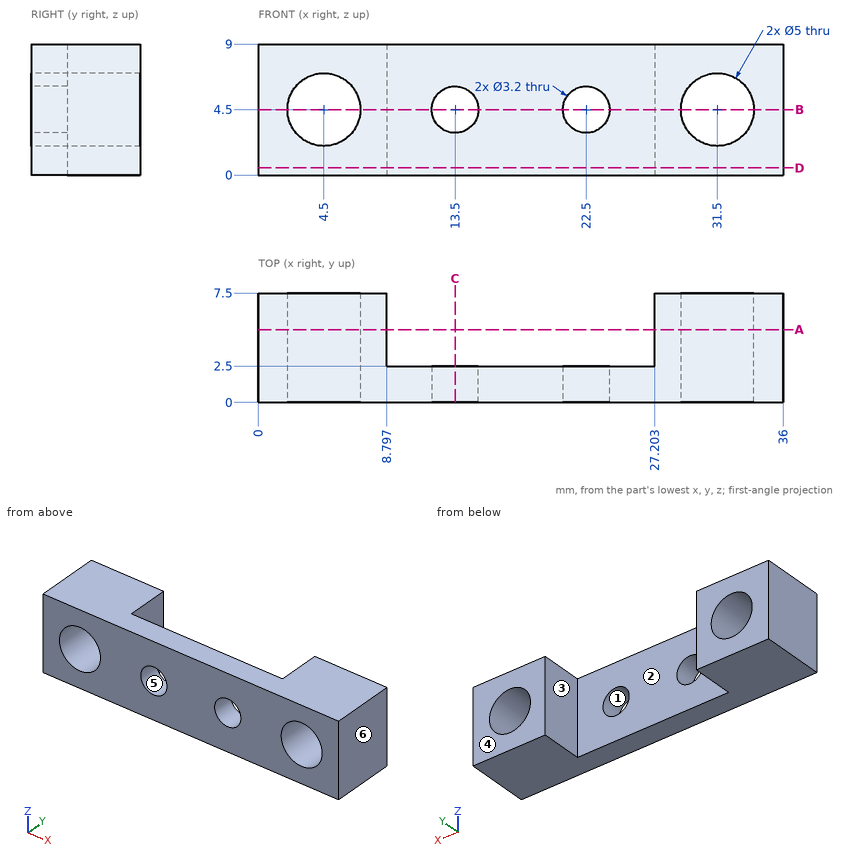
Answer from the drawing. Dimensions are ordinates in mm from the lowest x, y and z of the part. A direction names the side the tool comes from. Coordinates: 2 decimals unless noted, no trailing zeros. Order: outer loops, then holes, each group sorted by start corner. A loop starts at its lowest first (then second) coordinate and runs counter-clockwise, first axis right, second up. Notation, with made-up numbers: M 89,7 L 115,7 A12 cw 115,28 Z; hole C -11.75,-39.5 d6. An arc over 180 degrees is marked long. Put each result on its own line as item: value. Start each with the question number.
Item 1: Section C-C, the plane x = 13.5 is taken. Determine the outline of the cut face in (y, z), plus the area to 3 significant figures.
Item 2: Section D-D, the plane z = 0.5 is taken. Determine the outline of the cut face in (x, y).
Item 3: For the marked faces 1 and 2, determine the directions among +Z, -Z, +X, -X, +Y, -Y from which every point of the face is accessible in a straight line to the end or side of a thin tool.
Item 4: Consider probe 1 along X at (y, z) = (1.1, 4.5); probe 2 along X at (y, z) = (5, 1); probe 3 along X at (y, z) = (3.5, 6.25) (1 decimal). Determine where each line is inside the solid, lowest interval first. Write a range as [from, to].
Item 5: Section A-A, the plane y = 5 is taken. Determine the outline of the cut face in (x, z).
Item 6: The mould has two halves that part along X. Classify the marked faces 3, 4, 5 and 6: +X half, -X half, draft (parallel to the pull), parting line (faces both ways), or undercut.
Item 7: Section B-B, the plane z = 4.5 is taken. Determine the outline of the cut face in (x, y).
Item 8: Given pin 1 Ø5 at (x, z) = (13.5, 4.5) entering from +Y, flat-ended and moving along its own axis, determine where the tip first touches the part or whether it passes through.
Computed:
1. outline: M 0,0 L 2.5,0 L 2.5,2.9 L 0,2.9 Z; M 0,6.1 L 2.5,6.1 L 2.5,9 L 0,9 Z
1. area: 14.5 mm2
2. outline: M 0,0 L 36,0 L 36,7.5 L 27.2,7.5 L 27.2,2.5 L 8.8,2.5 L 8.8,7.5 L 0,7.5 Z
3. face 1: +Y, -Y
3. face 2: +Z, -Z, +Y
4. probe 1: x = [0, 2], [7, 11.9], [15.1, 20.9], [24.1, 29], [34, 36]
4. probe 2: x = [0, 8.8], [27.2, 36]
4. probe 3: x = [0, 2.7], [6.3, 8.8], [27.2, 29.7], [33.3, 36]
5. outline: M 0,0 L 8.8,0 L 8.8,9 L 0,9 Z; M 27.2,0 L 36,0 L 36,9 L 27.2,9 Z; hole C 4.5,4.5 d5; hole C 31.5,4.5 d5
6. face 3: undercut
6. face 4: draft
6. face 5: undercut
6. face 6: +X half
7. outline: M 0,0 L 2,0 L 2,7.5 L 0,7.5 Z; M 7,0 L 11.9,0 L 11.9,2.5 L 8.8,2.5 L 8.8,7.5 L 7,7.5 Z; M 15.1,0 L 20.9,0 L 20.9,2.5 L 15.1,2.5 Z; M 24.1,0 L 29,0 L 29,7.5 L 27.2,7.5 L 27.2,2.5 L 24.1,2.5 Z; M 34,0 L 36,0 L 36,7.5 L 34,7.5 Z
8. pin 1: stops at y = 2.5
